Can you work these out from the model? Positions are in its coordinate system, mm. Face numbers are marked on the shaded views. A direction names the side the tool comes from. Give positions to 0.01 mm unless a question says otherwise; leave off trailing zeros. Write each loop counter-clockwise with the first axis right and the second up, starting at its lowest first coordinate (ties: lowest second). Pieces come first, ordered by that corner, then holes. Notation, with made-up numbers: M 20.5,18 L 47.5,18 A18 cw 47.5,34 Z; hole C 63.25,71 d1. An arc over 180 degrees is marked long. Answer as CSV lines item,"result". Start each with the question number.
Autodesk Inventor part; units mm, degrees
ref_plane "Начальная плоскость" through (0, 0, 1.4142) normal (0, 0, 1) x (1, 0, 0)
ref_plane "Конечная плоскость" through (0, 0, 208.5858) normal (0, 0, 1) x (1, 0, 0)
ref_plane "РабПлоскость8" through (-0.7071, 0, 209.2929) normal (0.7071, 0, 0.7071) x (0.7071, 0, -0.7071)
ref_plane "Начальная плоскость" through (0, 0, 1.4142) normal (0, 0, 1) x (1, 0, 0)
ref_plane "Конечная плоскость" through (0, 0, 208.5858) normal (0, 0, 1) x (1, 0, 0)
sketch "Эскиз" plane through (0, 0, 0) normal (0, 0, 1) x (1, 0, 0)
  line L0 (36, -32.5) -> (0, -32.5)
  line L1 (36, -32.5) -> (36, -28.696)
  line L2 (33.6994, -26.2039) -> (9.9215, -24.3017)
  line L3 (4.4, -18.3208) -> (4.4, 18.3208)
  line L4 (33.6994, 26.2039) -> (9.9215, 24.3017)
  line L5 (36, 28.696) -> (36, 32.5)
  line L6 (0, 32.5) -> (36, 32.5)
  line L7 (0, -32.5) -> (0, 32.5)
  arc A0 (4.4, -18.3208) -> (9.9215, -24.3017) centre (10.4, -18.3208) ccw
  arc A1 (9.9215, 24.3017) -> (4.4, 18.3208) centre (10.4, 18.3208) ccw
  arc A2 (36, -28.696) -> (33.6994, -26.2039) centre (33.5, -28.696) ccw
  arc A3 (33.6994, 26.2039) -> (36, 28.696) centre (33.5, 28.696) ccw
  line L8 (0, 45.5) -> (0, -45.5) construction
  line L9 (-7.2974, 0) -> (43.7847, 0) construction
  point P0 (36, -26.388)
  point P1 (4.4, -23.86)
  point P2 (4.4, 23.86)
  point P3 (36, 26.388)
  dimension "d3" = 36
  dimension "d5" = 4.4
  dimension "d7" = 65
  dimension "d9" = 8.64
  dimension "d11" = 8.64
  dimension "d13" = 6.112
  dimension "d15" = 6.112
  dimension "d22" = 6
  dimension "d23" = 2.5
  dimension "d24" = 32.5
  dimension "d25" = 0
extrude "Тело" add sketch "Эскиз" along normal up to surface (207.1716 mm away) from surface at 1.4142
sketch "Sketch3" plane through (0, 0, 0) normal (0, 0, 1) x (1, 0, 0)
  line L0 (0, 0) -> (10, 0)
ref_plane "Work Plane7" through (0, 0, 0) normal (0, -1, 0) x (1, 0, 0)
sketch "Sketch4" plane through (0, 0, 0) normal (0, -1, 0) x (1, 0, 0)
  line L0 (-2, 1.4142) -> (12, 1.4142)
  line L1 (-2, 208.5858) -> (12, 208.5858)
  dimension "d29" = 207.1716
ref_plane "РабПлоскость8" through (-0.7071, 0, 209.2929) normal (0.7071, 0, 0.7071) x (0.7071, 0, -0.7071)
split "Разделение1" plane through (-0.7071, 0, 209.2929) removes the side toward (0.7071, 0, 0.7071)
ref_plane "РабПлоскость9" through (-0.7071, 0, 0.7071) normal (0.7071, 0, -0.7071) x (-0.7071, 0, -0.7071)
split "Разделение2" plane through (-0.7071, 0, 0.7071) removes the side toward (0.7071, 0, -0.7071)
equation "\"d3\" = b"
equation "\"d7\" = ParH"
equation "\"d22\" = R"
equation "\"d23\" = R1"
equation "\"d24\" = 0.5 * d7"
equation "\"d16\" = G_L"
equation "\"R1\" = 2.5"
equation "\"R\" = 6"
equation "\"t1\" = 4.4"
equation "\"t2\" = 7.2"
equation "\"ParH\" = 65"
equation "\"b\" = 36"
equation "\"msp_x1\" = 0.04 * b"
equation "\"msp_x2\" = -0.08 * t1 + 0.04 * b"
equation "\"G_L\" = d29"
equation "\"ex\" = 0"
equation "\"G_OFFSET_START\" = -1.41421"
equation "\"G_OFFSET_END\" = -1.41421"
equation "\"d26\" = -G_OFFSET_START"
equation "\"d27\" = G_OFFSET_END + B_L"
properties part number "Швеллер 6.5U-207,17 ГОСТ 8240-97" material "Сталь, мягкая, сварочная"
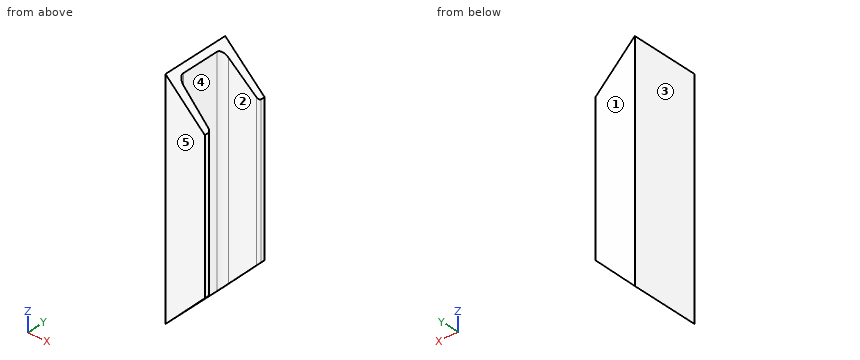
1) I want a section at D-D, the plane y = 3.5. Please give me the cut outline in (x, z).
2) I want a section at B-B, the plane z = 128.5. Please give me the cut outline in (x, y).
3) I need wall thicknesses on L1, parallel to X at y = -19, z = 30.5; L2, parallel to Y at x = 15, z = 162; L3, parallel to Y at x = 12, z = 166. Which ranges of each line are inside material? Lowest first, please. Write a range as from..to.
4) On a 3-axis mill with a long thin cutter (end or side, diameter ignored), from which of +Z, -Z, +X, -X, +Y, -Y can I reach the whole of each face in a straight line? I mean the marked faces 1 and 2. Say none if no direction works.
5) Thinking about a two-plate mould opening in Y: for the marked faces 3, 4 and 5, which applies, released by +Y, released by -Y, zero draft, split by the parting line, or undercut?
6) I'm going to push a flat-ended pin straight in: P1, Ø6, axis at y = -18.5, z = 23.5, coming from the +X side. Where does the tip first touch, or does it pass through?
7) I want a section at C-C, the plane x = 26. Please give me the cut outline in (y, z).
8) I want a section at A-A, the plane x = 14.5. Please give me the cut outline in (y, z), then the cut area to 3 significant figures.
Values found:
1,outline,"M 0,1.41 L 4.4,5.81 L 4.4,204.19 L 0,208.59 Z"
2,outline,"M 0,-32.5 L 36,-32.5 L 36,-28.7 A2.5 ccw 33.7,-26.2 L 9.92,-24.3 A6 cw 4.4,-18.32 L 4.4,18.32 A6 cw 9.92,24.3 L 33.7,26.2 A2.5 ccw 36,28.7 L 36,32.5 L 0,32.5 Z"
3,L1,"x = 0..4.44"
3,L2,"y = -32.5..-24.71, 24.71..32.5"
3,L3,"y = -32.5..-24.47, 24.47..32.5"
4,face 1,"+Z, -Z, +X, -X, +Y"
4,face 2,"+Z, -Z, +X"
5,face 3,"zero draft"
5,face 4,"undercut"
5,face 5,"released by -Y"
6,P1,"stops at x = 5.31"
7,outline,"M -32.5,27.41 L -25.59,27.41 L -25.59,182.59 L -32.5,182.59 Z; M 25.59,27.41 L 32.5,27.41 L 32.5,182.59 L 25.59,182.59 Z"
8,outline,"M -32.5,15.91 L -24.67,15.91 L -24.67,194.09 L -32.5,194.09 Z; M 24.67,15.91 L 32.5,15.91 L 32.5,194.09 L 24.67,194.09 Z"
8,area,"2,790 mm²"
